Read the model definition and answer for the solid it produces. Units are mm, in the model's axes. Face numbers are marked on the shaded views. A direction names the side the tool comes from. Coordinates: 2 decimals unless noted, no trailing zeros. Write each loop counter-clockwise with the first axis right and the second up, starting at its lowest first coordinate (ties: lowest second). Pieces come first, ordered by that corner, then holes. Notation, with made-up numbers: (82, 28.5) - (99, 28.5) arc R27 ccw to (99, 48.5) - close; hole circle Ø7 at (61, -16). An arc over 180 degrees is marked (long way). Use a Markdown table: item, result.
from build123d import *

# Parameters (mm, degrees)
SKETCH_R          = 16.3
SKETCH_R_2        = 15.05
PAD_DEPTH         = 7
SKETCH001_W       = 35.5
SKETCH001_H       = 35.5
SKETCH001_R       = 12.55
PAD001_DEPTH      = 2
SKETCH002_W       = 5.6
SKETCH002_H       = 2
POCKET_DEPTH      = 25
POCKET_DEPTH_BACK = 25
FILLET002_R       = 0.5
FILLET003_R       = 0.5
FILLET004_R       = 0.5


with BuildPart() as part:
    # Sketch → Pad (new body)
    with BuildSketch(Plane.XZ):
        Circle(SKETCH_R)
        Circle(SKETCH_R_2, mode=Mode.SUBTRACT)
    extrude(amount=PAD_DEPTH)

    # Sketch001 → Pad001 (join)
    with BuildSketch(Plane.XZ):
        Rectangle(SKETCH001_W, SKETCH001_H)
        Circle(SKETCH001_R, mode=Mode.SUBTRACT)
    extrude(amount=-PAD001_DEPTH)

    # Sketch002 (on DatumPlane) → Pocket (cut, two sides)
    with BuildSketch(Plane.YZ) as pocket_sk:
        with Locations((-4.2, 0)):
            Rectangle(SKETCH002_W, SKETCH002_H)
    extrude(amount=-POCKET_DEPTH, mode=Mode.SUBTRACT)
    extrude(pocket_sk.sketch, amount=POCKET_DEPTH_BACK, mode=Mode.SUBTRACT)

    # Fillet002
    fillet002_edges = [part.edges().sort_by_distance(p)[0] for p in [
        (-17.75, 1, -17.75),
        (-17.75, 1, 17.75),
    ]]
    fillet(fillet002_edges, radius=FILLET002_R)

    # Fillet003
    fillet003_edges = [part.edges().sort_by_distance(p)[0] for p in [
        (-17.75, 0, 0),
        (0.25, 0, 17.75),
        (0.25, 0, -17.75),
        (17.75, 0, 0),
    ]]
    fillet(fillet003_edges, radius=FILLET003_R)

    # Fillet004
    fillet004_edges = [part.edges().sort_by_distance(p)[0] for p in [
        (0, -7, 15.05),
        (0, -7, 16.3),
        (0, -7, -16.3),
        (0, -7, -15.05),
    ]]
    fillet(fillet004_edges, radius=FILLET004_R)


with BuildPart() as part_1:
    # Body placement: moved
    add(part.part.moved(Location((0, -3, 0))))


solid = part_1.part
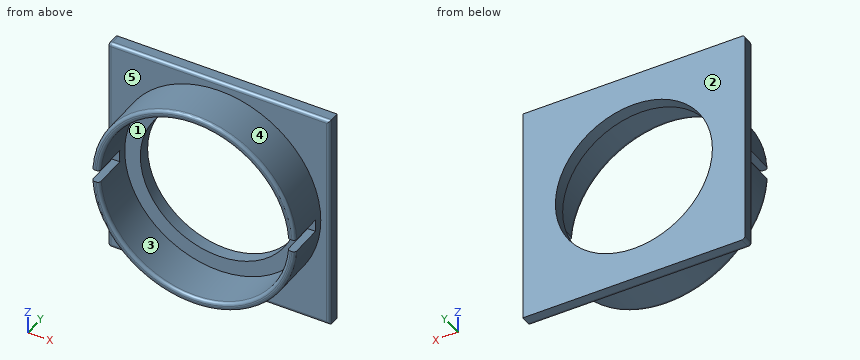
(1) Straight lines are drawn through the part: L1, parallel to Z at x = 0, y = -2.4; L2, parallel to Z at x = 0, y = -8; L3, parallel to Y at x = -7, z = 15. For each, find the intervals that lie inside material, in ascending order.
Report:
| item | result |
|---|---|
| L1 | z = -17.75 to -12.55, 12.55 to 17.75 |
| L2 | z = -16.3 to -15.05, 15.05 to 16.3 |
| L3 | y = -3 to -1 |
(2) A cutting plane is placed at B-B, the plane x = 0. Write down the section's boundary in (y, z), and give its area (3 significant figures).
Report:
| item | result |
|---|---|
| outline | (-10, -15.8) arc R0.5 ccw to (-9.5, -16.3) - (-3, -16.3) - (-3, -17.25) arc R0.5 ccw to (-2.5, -17.75) - (-1, -17.75) - (-1, -12.55) - (-3, -12.55) - (-3, -15.05) - (-9.5, -15.05) arc R0.5 ccw to (-10, -15.55) - close; (-10, 15.55) arc R0.5 ccw to (-9.5, 15.05) - (-3, 15.05) - (-3, 12.55) - (-1, 12.55) - (-1, 17.75) - (-2.5, 17.75) arc R0.5 ccw to (-3, 17.25) - (-3, 16.3) - (-9.5, 16.3) arc R0.5 ccw to (-10, 15.8) - close |
| area | 38.0 mm² |
(3) Each of these flat-tipped pins is pushed along its axis until it touches: P1, Ø2, axis at x = 4, y = -7, coming from the +Z side; P2, Ø1.4, axis at x = 15.5, y = -8, coming from the -Z side; P3, Ø3, axis at y = -7.5, z = -10.5, coming from the -X side. Where does it stop, or does it pass through?
Report:
| item | result |
|---|---|
| P1 | stops at z = 16.02 |
| P2 | stops at z = -6.83 |
| P3 | stops at x = -13.59 |
(4) The mould has two halves that part along X. Classify the marked faces 3, 4 and 5: pulls with the +X half, pulls with the -X half, needs draft (parallel to the pull), parting line crosses it, or undercut.
Report:
| item | result |
|---|---|
| face 3 | undercut |
| face 4 | parting line crosses it |
| face 5 | needs draft |
(5) A cutting plane is placed at A-A, the plane z = 0. Write down the section's boundary in (x, y), and give its area (3 significant figures).
Report:
| item | result |
|---|---|
| outline | (-17.75, -2.5) arc R0.5 ccw to (-17.25, -3) - (-16.3, -3) - (-16.3, -4.4) - (-15.05, -4.4) - (-15.05, -3) - (-12.55, -3) - (-12.55, -1) - (-17.75, -1) - close; (12.55, -3) - (15.05, -3) - (15.05, -4.4) - (16.3, -4.4) - (16.3, -3) - (17.25, -3) arc R0.5 ccw to (17.75, -2.5) - (17.75, -1) - (12.55, -1) - close |
| area | 24.2 mm² |
(6) For the marked faces 1 and 2, determine the directions among +Z, -Z, +X, -X, +Y, -Y from which every point of the face is accessible in a straight line to the end or side of a thin tool.
Report:
| item | result |
|---|---|
| face 1 | -Y |
| face 2 | +Z, -Z, +X, -X, +Y |
(7) A cutting plane is placed at C-C, the plane y = -7.25. Write down the section's boundary in (x, z), and give its area (3 significant figures).
Report:
| item | result |
|---|---|
| outline | (-16.27, -1) arc R16.3 ccw to (16.27, -1) - (15.02, -1) arc R15.05 cw to (-15.02, -1) - close; (-16.27, 1) - (-15.02, 1) arc R15.05 cw to (15.02, 1) - (16.27, 1) arc R16.3 ccw to start |
| area | 118 mm² |
